from build123d import *

# Parameters (mm, degrees)
SKETCH_1_R               = 13.5
EXTRUDE_1_DEPTH          = 6
EXTRUDE_START            = -6
EXTRUDE_2_DEPTH          = 6
EXTRUDE_3_DEPTH          = 21
SKETCH_5_R               = 3.5
CUT_EXTRUDE_1_DEPTH      = 41.943558712
CUT_EXTRUDE_3_DEPTH      = 49.849257927
CUT_EXTRUDE_3_DEPTH_BACK = 49.849257927
FILLET_3_R               = 10


with BuildPart() as part:
    # 草图1 → 凸台-拉伸1 (new body)
    with BuildSketch(Plane.XY):
        Circle(SKETCH_1_R)
        Polygon((10.35, 0), (7.318555185, -7.318555185), (0, -10.35), (-7.318555185, -7.318555185), (-10.35, 0), (-7.318555185, 7.318555185), (0, 10.35), (7.318555185, 7.318555185), align=None, mode=Mode.SUBTRACT)
    extrude(amount=EXTRUDE_1_DEPTH)

    # 草图2 → 凸台-拉伸2 (add)
    with BuildSketch(Plane.XY.offset(6).offset(EXTRUDE_START)):
        with BuildLine():
            Line((-10.5, -8.485281374), (-10.5, -30))
            Line((-10.5, -30), (10.5, -30))
            Line((10.5, -30), (10.5, -8.485281374))
            ThreePointArc((10.5, -8.485281374), (0, -13.5), (-10.5, -8.485281374))
        make_face()
    extrude(amount=EXTRUDE_2_DEPTH)

    # 草图4 → 凸台-拉伸3 (add)
    with BuildSketch(Plane(origin=(10.5, 0, 0), x_dir=(0, 0, -1), z_dir=(1, 0, 0))):
        Polygon((-6, -27.257359313), (-14.5, -35.757359313), (-10.257359313, -40), (0, -29.742640687), align=None)
    extrude(amount=-EXTRUDE_3_DEPTH)

    # 草图5 → 切除-拉伸1 (cut, through all)
    with BuildSketch(Plane(origin=(0, -10.628679656, -10.628679656), x_dir=(1, 0, 0), z_dir=(0, 0.7071067811865436, 0.7071067811865515))):
        with Locations(Location((0, -29.537319575, 0), (0, 0, 270))):
            Circle(SKETCH_5_R)
    extrude(amount=-CUT_EXTRUDE_1_DEPTH, mode=Mode.SUBTRACT)

    # 草图6 → 切除-拉伸3 (cut, two sides: drawn at the far end of the back side and taken through both)
    with BuildSketch(Plane(origin=(10.5, 0, 0), x_dir=(0, 0, -1), z_dir=(1, 0, 0)).offset(-CUT_EXTRUDE_3_DEPTH_BACK)):
        Polygon((0, -29.742640687), (-0.257359313, -30), (0, -30), align=None)
    extrude(amount=CUT_EXTRUDE_3_DEPTH + CUT_EXTRUDE_3_DEPTH_BACK, mode=Mode.SUBTRACT)

    # 圆角3
    fillet_3_edges = [part.edges().sort_by_distance(p)[0] for p in [
        (-10.5, -8.485281374, 3),
        (10.5, -8.485281374, 3),
        (-10.5, -37.878679656, 12.378679656),
        (10.5, -37.878679656, 12.378679656),
    ]]
    fillet(fillet_3_edges, radius=FILLET_3_R)


solid = part.part
Could you check a few things on this model? Use its own coordinates, in mm. A direction names the side the tool comes from. Round coordinates to 2 decimals unless told otherwise and drop trailing zeros. Write each loop counter-clockwise with the first axis right and the second up, starting at its lowest first coordinate (ties: lowest second). Pieces come first, ordered by that corner, then holes. Notation, with made-up numbers: (55, -33.5) - (87, -33.5) arc R35 cw to (87, 0.5) - close; hole circle Ø10 at (71.5, -7.5). An arc over 180 degrees is marked (long way). Use a Markdown table: item, result.
Q1. Please list where these lines run through material, in increasing order: L1, parallel to X at y = -21.5, z = 2.75; L2, parallel to Z at x = -10, y = -23.5; L3, parallel to Y at x = -8.5, z = 2.5.
Output values:
| item | result |
|---|---|
| L1 | -10.5 to 10.5 |
| L2 | 0 to 6 |
| L3 | -32.24 to -4.47, 4.47 to 10.49 |
Q2. I want a section at C-C (x = 9). List the corners of the cut face in (y, z) for me.
Output values:
| item | result |
|---|---|
| outline | (-36.65, 6.91) - (-29.74, 0) - (-3.26, 0) - (-3.26, 6) - (-27.26, 6) - (-32.41, 11.15) - close; (3.26, 0) - (10.06, 0) - (10.06, 6) - (3.26, 6) - close |
Q3. Thinking about a two-plate mould opening in X: for faces 1 (the flat face through (0.01, -37.85, 12.41)), 2 (the flat face through (-8.813, -3.711, 2.958)), 3 (the cylindrical face through (-7.493, -35.892, 10.333)), which applies, released by +X, released by -X, zero draft, split by the parting line, or undercut?
Output values:
| item | result |
|---|---|
| face 1 | zero draft |
| face 2 | undercut |
| face 3 | released by -X |
Q4. For pin 1 (8 mm diameter, centred on y = -15, z = 5, fed in from -X); pin 2 (3 mm diameter, centred on x = 5.5, z = 7, fed in from +Y); pin 3 (3 mm diameter, centred on x = 5, y = -4, fed in from -Z); pin 4 (6 mm diameter, centred on x = -7, z = 12, fed in from -Y), each with a flat end and sliding along its axis, tell me the tip position at first contact or that it passes through.
Output values:
| item | result |
|---|---|
| pin 1 | x = -10.51 |
| pin 2 | y = 12.77 |
| pin 3 | through |
| pin 4 | y = -39 |
Q5. For faces 4 (the flat face through (10.5, -22, 3)), 5 (the flat face through (-10.5, -22, 3)), 6 (the flat face through (0, -11, 6)), 7 (the flat face through (-3.608, -8.855, 2.958)), 8 (the cylindrical face through (1.051, -35.967, 10.526)), which set-ups out of +Z, -Z, +X, -X, +Y, -Y let a thin tool reach every point of the face, with its end or its side?
Output values:
| item | result |
|---|---|
| face 4 | +Z, -Z, +X, -Y |
| face 5 | +Z, -Z, -X, -Y |
| face 6 | +Z, +X, -X, +Y |
| face 7 | +Z, -Z |
| face 8 | none |
Q6. I want a section at D-D (z = 2). List the corners of the cut face in (x, y) for me, plus the area to 3 significant figures.
Output values:
| item | result |
|---|---|
| outline | (-11.78, -6.6) arc R10 cw to (-10.5, -11.49) - (-10.5, -31.74) - (10.5, -31.74) - (10.5, -11.49) arc R10 cw to (11.78, -6.6) arc R13.5 ccw (long way) to start; hole (-10.35, 0) - (-7.32, -7.32) - (0, -10.35) - (7.32, -7.32) - (10.35, 0) - (7.32, 7.32) - (0, 10.35) - (-7.32, 7.32) - close |
| area | 686 mm2 |
Q7. I want a section at A-A (y = 2.5). List the corners of the cut face in (x, z) for me, plus the area to 3 significant figures.
Output values:
| item | result |
|---|---|
| outline | (-13.27, 0) - (-9.31, 0) - (-9.31, 6) - (-13.27, 6) - close; (9.31, 0) - (13.27, 0) - (13.27, 6) - (9.31, 6) - close |
| area | 47.4 mm2 |
Q8. I want a section at B-B (x = -2.75). List the corners of the cut face in (y, z) for me.
Output values:
| item | result |
|---|---|
| outline | (-39.82, 10.08) - (-37.29, 7.55) - (-33.05, 11.79) - (-35.58, 14.32) - close; (-34.23, 4.48) - (-29.74, 0) - (-9.21, 0) - (-9.21, 6) - (-27.26, 6) - (-29.98, 8.73) - close; (9.21, 0) - (13.22, 0) - (13.22, 6) - (9.21, 6) - close |
